Can you work these out from the model? Positions are in its coordinate system, mm. A direction names the side the tool comes from. Coordinates: 2 decimals unless noted, no trailing zeros. Order: outer loops, then holes, each group sorted by start corner. A loop starts at its lowest first (then second) coordinate and runs counter-clockwise, first axis right, second up. Notation, with made-up numbers: M 88.25,-3 L 116.25,-3 A14 ccw 116.25,9 Z; hole C 8,35 d9. An arc over 180 degrees is marked long. Answer as CSV lines item,"result". Start each with the question number.
1. Will this pin go through, and if not, where does the flat tip stop? pin 1 (1.5 mm diameter, centred on x = 5, y = 96.5, fed in from -Z).
2. If we mould it in two halves opening along Y, with no side actions, what happens to faces 3 (the face through (-25.4, -2, 3)), 4 (the face through (0, -123.825, 3)), 5 (the face through (0, -152.4, 3)), 6 (the face through (0, 152.4, 3))? For each: released by +Y, released by -Y, zero draft, split by the parting line, or undercut.
3. On a 3-axis mill with a long thin cutter (end or side, diameter ignored), from which of +Z, -Z, +X, -X, +Y, -Y can I reach the whole of each face in a straight line? I mean faces 1 (the face through (0, 2, 0)), 2 (the face through (15.874, -127.07, 3.131)). Say none if no direction works.
4. I need wall thicknesses on line 1 along Y through (x, z) = (5, 1.25) (3 decimals); line 2 along Y through (x, z) = (-14.5, 0.5). Which ranges of each line are inside material? Lowest first, please. Write a range as from..to.
5. If we section it at B-B (z = 3.5): List the corners of the cut face in (x, y) for me (3 decimals).
6. If we section it at A-A (y = -127): List the corners of the cut face in (x, z) for me (3 decimals).
```python
from build123d import *

# Parameters (mm, degrees)
F0_W     = 50.8
F0_H     = 304.8
F1_DEPTH = 6.35
F3_DEPTH = 25.4


with BuildPart() as f1:
    # F0 (on Top) → F1 (new body)
    with BuildSketch(Plane.XY):
        Rectangle(F0_W, F0_H)
    extrude(amount=F1_DEPTH)

    # F2 (on Top) → F3 (cut)
    with BuildSketch(Plane.XY):
        with BuildLine():
            Line((12.7, 130.175), (-12.7, 130.175))
            ThreePointArc((-12.7, 130.175), (-15.875, 127), (-12.7, 123.825))
            Line((-12.7, 123.825), (12.7, 123.825))
            ThreePointArc((12.7, 123.825), (15.875, 127), (12.7, 130.175))
        make_face()
        with BuildLine():
            Line((12.7, -123.825), (-12.7, -123.825))
            ThreePointArc((-12.7, -123.825), (-15.875, -127), (-12.7, -130.175))
            Line((-12.7, -130.175), (12.7, -130.175))
            ThreePointArc((12.7, -130.175), (15.875, -127), (12.7, -123.825))
        make_face()
    extrude(amount=F3_DEPTH, mode=Mode.SUBTRACT)


solid = f1.part
```
Solved:
1,pin 1,"z = 0"
2,face 3,"zero draft"
2,face 4,"undercut"
2,face 5,"released by -Y"
2,face 6,"released by +Y"
3,face 1,"-Z, +X, -X, +Y, -Y"
3,face 2,"+Z, -Z"
4,line 1,"-152.4..-130.175, -123.825..123.825, 130.175..152.4"
4,line 2,"-152.4..-129.62, -124.38..124.38, 129.62..152.4"
5,outline,"M -25.4,-152.4 L 25.4,-152.4 L 25.4,152.4 L -25.4,152.4 Z; hole M -12.7,-130.175 L 12.7,-130.175 A3.175 ccw 12.7,-123.825 L -12.7,-123.825 A3.175 ccw Z; hole M -12.7,123.825 L 12.7,123.825 A3.175 ccw 12.7,130.175 L -12.7,130.175 A3.175 ccw Z"
6,outline,"M -25.4,0 L -15.875,0 L -15.875,6.35 L -25.4,6.35 Z; M 15.875,0 L 25.4,0 L 25.4,6.35 L 15.875,6.35 Z"
